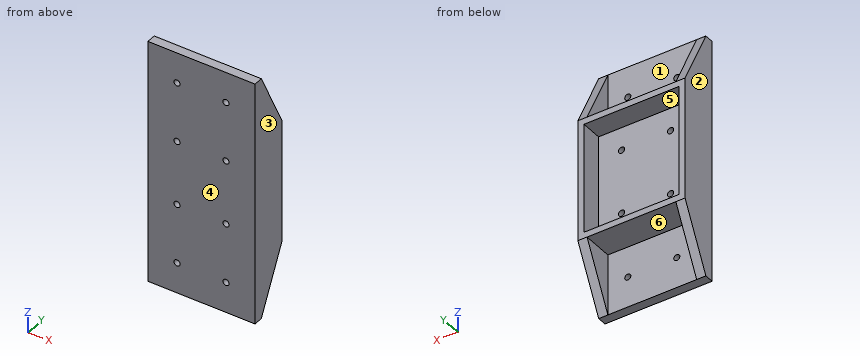
from build123d import *

# Parameters (mm, degrees)
SKETCH1_W           = 35
SKETCH1_H           = 40
BOSS_EXTRUDE1_DEPTH = 10
SKETCH2_W           = 31
SKETCH2_H           = 36
CUT_EXTRUDE1_DEPTH  = 7
SKETCH3_W           = 35
SKETCH3_H           = 80
BOSS_EXTRUDE2_DEPTH = 3
BOSS_EXTRUDE3_DEPTH = 3
SKETCH6_R           = 1
CUT_EXTRUDE2_DEPTH  = 6
SKETCH7_R           = 1
CUT_EXTRUDE3_DEPTH  = 3


with BuildPart() as part:
    # Sketch1 → Boss-Extrude1 (new body)
    with BuildSketch(Plane(origin=(0, 0, 0), x_dir=(1, 0, 0), z_dir=(0, 1, 0))):
        Rectangle(SKETCH1_W, SKETCH1_H)
    extrude(amount=BOSS_EXTRUDE1_DEPTH)

    # Sketch2 → Cut-Extrude1 (cut)
    with BuildSketch(Plane(origin=(0, 10, 0), x_dir=(1, 0, 0), z_dir=(0, 1, 0))):
        Rectangle(SKETCH2_W, SKETCH2_H)
    extrude(amount=-CUT_EXTRUDE1_DEPTH, mode=Mode.SUBTRACT)

    # Sketch3 → Boss-Extrude2 (add)
    with BuildSketch(Plane.XZ):
        Rectangle(SKETCH3_W, SKETCH3_H)
    extrude(amount=BOSS_EXTRUDE2_DEPTH)

    # Sketch5 → Boss-Extrude3 (add)
    with BuildSketch(Plane.ZY.offset(17.5)):
        Polygon((-20, 10), (-20, 0), (-40, 0), align=None)
        Polygon((20, 10), (20, 0), (40, 0), align=None)
    boss_extrude3 = extrude(amount=-BOSS_EXTRUDE3_DEPTH)

    # Mirror1: Boss-Extrude3 across plane
    add(boss_extrude3.mirror(Plane(origin=(0, 0, 0), x_dir=(0, 0, 1), z_dir=(1, 0, 0))))

    # Sketch6 → Cut-Extrude2 (cut)
    with BuildSketch(Plane(origin=(0, 3, 0), x_dir=(1, 0, 0), z_dir=(0, 1, 0))):
        with Locations(Location((-8, 10.5, 0), (0, 0, 270))):
            Circle(SKETCH6_R)
        with Locations(Location((8, 10.5, 0), (0, 0, 270))):
            Circle(SKETCH6_R)
        with Locations(Location((-8, -10.5, 0), (0, 0, 270))):
            Circle(SKETCH6_R)
        with Locations(Location((8, -10.5, 0), (0, 0, 270))):
            Circle(SKETCH6_R)
    extrude(amount=-CUT_EXTRUDE2_DEPTH, mode=Mode.SUBTRACT)

    # Sketch7 → Cut-Extrude3 (cut)
    with BuildSketch(Plane(origin=(0, 0, 0), x_dir=(1, 0, 0), z_dir=(0, 1, 0))):
        with Locations(Location((-8, 30, 0), (0, 0, 270))):
            Circle(SKETCH7_R)
        with Locations(Location((8, 30, 0), (0, 0, 270))):
            Circle(SKETCH7_R)
    cut_extrude3 = extrude(amount=-CUT_EXTRUDE3_DEPTH, mode=Mode.SUBTRACT)

    # Mirror2: Cut-Extrude3 across plane
    add(cut_extrude3.mirror(Plane.XY), mode=Mode.SUBTRACT)


solid = part.part
Source: CAD feature listing. Evaluate the final solid. Frame: model axes, mm. Face numbers are marked on the shaded views. A direction names the side the tool comes from. Give positions to 0.01 mm unless a question says otherwise; leave off trailing zeros. Write each loop counter-clockwise with the first axis right and the second up, starting at its lowest first coordinate (ties: lowest second). Pieces come first, ordered by that corner, then holes. Notation, with made-up numbers: (86, -19) - (136, -19) arc R5 cw to (136, -12) - close; hole circle Ø6 at (2, 67). An arc over 180 degrees is marked (long way). Write item = value, one per line. Start each with the question number.
Q1. Draft query along X for the marked faces 1, 2 and 3. Return one class per face: +X half, -X half, draft (parallel to the pull), parting line (faces both ways), or undercut.
Q2. Pin query (flat end, axial travel): pin 1 Ø4 at (x, y) = (13.5, 7.5) entering from -Z; pin 2 Ø1.5 at (x, y) = (-3, 1) entering from +Z; pin 3 Ø2 at (x, y) = (1.5, 6) entering from -Z. Return the tip coordinate at first contact, or that it passes through.
Q3. Material intervals for probe 1 along X at (y, z) = (-1.1, -10.5); probe 2 along X at (y, z) = (2.5, 23); probe 3 along X at (y, z) = (4.5, -8), sorted ascending.
Q4. Cut plane C-C, the plane y = 6. Return loops of the section in (x, z).
Q5. Cut plane A-A, the plane x = 8. Return loops of the section in (y, z).
Q6. Cut plane D-D, the plane y = 1.25. Return loops of the section in (x, z), then the cut area to 3 significant figures.
Q7. Reachability of the marked faces 4, 5 and 6 from +Z, -Z, +X, -X, +Y, -Y: full face, straight path, thin tool, end or side. Return the list, or none.
Q8. Cut plane B-B, the plane z = 30. Return loops of the section in (x, y), then the cut area to 3 significant figures.
Computed values:
q1.face_1 = undercut
q1.face_2 = -X half
q1.face_3 = +X half
q2.pin_1 = -28.46
q2.pin_2 = 20
q2.pin_3 = -20
q3.probe_1 = -17.5 to -9, -7 to 7, 9 to 17.5
q3.probe_2 = -17.5 to -14.5, 14.5 to 17.5
q3.probe_3 = -17.5 to -15.5, 15.5 to 17.5
q4.outline = (-17.5, -28) - (-14.5, -28) - (-14.5, -20) - (14.5, -20) - (14.5, -28) - (17.5, -28) - (17.5, 28) - (14.5, 28) - (14.5, 20) - (-14.5, 20) - (-14.5, 28) - (-17.5, 28) - close; hole (-15.5, -18) - (15.5, -18) - (15.5, 18) - (-15.5, 18) - close
q5.outline = (-3, -40) - (0, -40) - (0, -31) - (-3, -31) - close; (-3, -29) - (0, -29) - (0, -20) - (10, -20) - (10, -18) - (3, -18) - (3, -11.5) - (-3, -11.5) - close; (-3, -9.5) - (3, -9.5) - (3, 9.5) - (-3, 9.5) - close; (-3, 11.5) - (3, 11.5) - (3, 18) - (10, 18) - (10, 20) - (0, 20) - (0, 29) - (-3, 29) - close; (-3, 31) - (0, 31) - (0, 40) - (-3, 40) - close
q6.outline = (-17.5, -37.5) - (-14.5, -37.5) - (-14.5, -20) - (14.5, -20) - (14.5, -37.5) - (17.5, -37.5) - (17.5, 37.5) - (14.5, 37.5) - (14.5, 20) - (-14.5, 20) - (-14.5, 37.5) - (-17.5, 37.5) - close; hole circle Ø2 at (-8, -10.5); hole circle Ø2 at (-8, 10.5); hole circle Ø2 at (8, -10.5); hole circle Ø2 at (8, 10.5)
q6.area = 1,600 mm²
q7.face_4 = +Z, -Z, +X, -X, -Y
q7.face_5 = +Y
q7.face_6 = -Z, +Y
q8.outline = (-17.5, -3) - (-9, -3) - (-9, 0) - (-14.5, 0) - (-14.5, 5) - (-17.5, 5) - close; (-7, -3) - (7, -3) - (7, 0) - (-7, 0) - close; (9, -3) - (17.5, -3) - (17.5, 5) - (14.5, 5) - (14.5, 0) - (9, 0) - close
q8.area = 123 mm²
